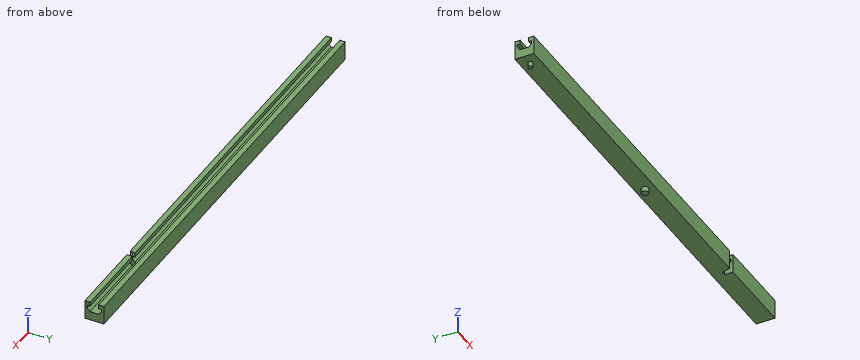
Autodesk Inventor part; units mm, degrees
ref_plane "YZ Plane" through (0, 0, 0) normal (1, 0, 0) x (0, 1, 0)
ref_plane "XZ Plane" through (0, 0, 0) normal (0, 1, 0) x (-1, 0, 0)
ref_plane "XY Plane" through (0, 0, 0) normal (0, 0, 1) x (1, 0, 0)
sketch "Sketch1" plane through (0, 0, 0) normal (0, 0, 1) x (1, 0, 0)
  line L0 (-600, -25) -> (600, -25)
  line L1 (600, -25) -> (600, 25)
  line L2 (600, 25) -> (-600, 25)
  line L3 (-600, 25) -> (-600, -25)
  line L4 (-600, -25) -> (600, 25) construction
  line L5 (600, -25) -> (-600, 25) construction
  point P0 (0, 0)
  dimension "d0" = 1200
  dimension "d1" = 50
extrude "Extrusion1" add sketch "Sketch1" along normal blind 50
sketch "Sketch2" plane through (0, 0, 0) normal (0, 0, -1) x (-1, 0, 0)
  circle A0 centre (0, 0) radius 9
  circle A1 centre (570, 0) radius 6
  line L0 (600, 25) -> (600, -25)
  line L1 (-600, 25) -> (600, 25)
  dimension "d13" = 18
  dimension "d20" = 30
  dimension "d21" = 12
  dimension "d22" = 50
  dimension "d23" = 25
extrude "Extrusion2" add sketch "Sketch2" along normal blind 13
sketch "Sketch5" plane through (0, 0, 0) normal (0, 0, -1) x (-1, 0, 0)
  line L0 (600, -25) -> (-600, -25)
  line L1 (-391, -25) -> (-391, -3)
  line L2 (-391, -3) -> (-380, -3)
  line L3 (-380, -3) -> (-380, -25) construction
  line L4 (-380, -3) -> (-374.1051, -25)
  point P0 (0, 0)
  dimension "d30" = 15
  dimension "d31" = 22
  dimension "d32" = 11
  dimension "d33" = 209
extrude "Extrusion4" cut sketch "Sketch5" against normal through all
sketch "Sketch6" plane through (600, -25, 0) normal (1, 0, 0) x (0, 0, -1)
  line L0 (-50, 0) -> (-50, 50)
  line L1 (0, 50) -> (-50, 50)
  line L2 (0, 0) -> (0, 50)
  line L3 (0, 50) -> (-50, 50)
  line L4 (-50, 0) -> (-50, 50)
  line L5 (0, 0) -> (-50, 0)
  line L6 (-50, 36) -> (-39, 36)
  line L7 (-39, 36) -> (-39, 44)
  line L8 (-50, 14) -> (-39, 14)
  line L9 (-39, 14) -> (-39, 6)
  line L10 (-23, 36.8677) -> (-23, 13.1323)
  line L11 (-23, 36.8677) -> (-31.5, 44)
  line L12 (-31.5, 44) -> (-39, 44)
  line L13 (-23, 13.1323) -> (-31.5, 6)
  line L14 (-31.5, 6) -> (-39, 6)
  point P0 (0, 25)
  dimension "d36" = 14
  dimension "d37" = 14
  dimension "d38" = 8
  dimension "d42" = 16
  dimension "d43" = 11
  dimension "d44" = 7.5
  dimension "d88" = 140
  dimension "d89" = 140
extrude "Extrusion5" cut sketch "Sketch6" against normal through all contours L0 L6 L7 L12 L11 L10 L13 L14 L9 L8
equation "\"d23\" = 0.5 * d22"
equation "\"d37\" = d36"
equation "\"d89\" = d88"
properties part number "u_lange_Stange" material "Birch"
Here's how the part is built. I have some questions about the finished solid (model axes, mm). Coordinates: 2 decimals unless noted, no trailing zeros. Write each loop counter-clockwise with the first axis right and the second up, starting at its lowest first coordinate (ties: lowest second). Pieces come first, ordered by that corner, then holes. Notation, with made-up numbers: M 34.25,38 L 38.25,38 A26 cw 38.25,68 Z; hole C 20.25,25.5 d5. An arc over 180 degrees is marked long. Answer as CSV lines item,"result". Start each with the question number.
Q1. Will these pins go through, and if not, where does the flat tip stop? pin 1 Ø12 at (x, z) = (388, 16.5) entering from -Y; pin 2 Ø9 at (x, y) = (-275.5, 14) entering from -Z; pin 3 Ø3 at (x, z) = (218.5, -2.5) entering from +Y; pin 4 Ø7 at (x, y) = (-201, 0.5) entering from +Z.
Q2. Suppose I cut it at A-A, the plane x = -67.5. List the corners of the cut face in (y, z) for me.
Q3. I need wall thicknesses on probe 1 along Y at (x, z) = (-103, 45); probe 2 along Y at (x, z) = (-337, 32); probe 3 along Z at (x, y) = (-246, -12). Which ranges of each line are inside material? Lowest first, please. Write a range as [from, to].
Entries:
1,pin 1,"stops at y = -25"
1,pin 2,"stops at z = 0"
1,pin 3,"passes through"
1,pin 4,"stops at z = 23"
2,outline,"M -25,0 L 25,0 L 25,50 L 11,50 L 11,39 L 19,39 L 19,31.5 L 11.87,23 L -11.87,23 L -19,31.5 L -19,39 L -11,39 L -11,50 L -25,50 Z"
3,probe 1,"y = [-25, -11], [11, 25]"
3,probe 2,"y = [-25, -19], [19, 25]"
3,probe 3,"z = [0, 23.16], [39, 50]"
